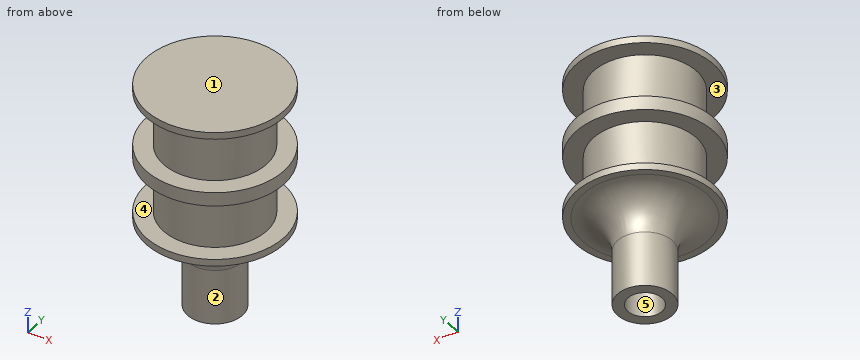
```python
from build123d import *

# Parameters (mm, degrees)
CROQUIS1_R              = 10
SALIENTE_EXTRUIR1_DEPTH = 5
CROQUIS2_R              = 10
CROQUIS2_R_2            = 7.5
CORTAR_EXTRUIR1_DEPTH   = 4
CROQUIS3_R              = 4
SALIENTE_EXTRUIR2_DEPTH = 13
CROQUIS4_R              = 2.5
CORTAR_EXTRUIR2_DEPTH   = 8
REDONDEO1_R             = 5


with BuildPart() as part:
    # Croquis1 → Saliente-Extruir1 (new, symmetric)
    with BuildSketch(Plane(origin=(0, 0, 0), x_dir=(0, 1, 0), z_dir=(0, 0, 1))):
        with Locations(Location((0, 0, 0), (0, 0, 270))):
            Circle(CROQUIS1_R)
    extrude(amount=SALIENTE_EXTRUIR1_DEPTH, both=True)

    # Croquis2 → Cortar-Extruir1 (cut, symmetric)
    with BuildSketch(Plane(origin=(0, 0, 0), x_dir=(0, 1, 0), z_dir=(0, 0, 1))):
        with Locations(Location((0, 0, 0), (0, 0, 270))):
            Circle(CROQUIS2_R)
        with Locations(Location((0, 0, 0), (0, 0, 270))):
            Circle(CROQUIS2_R_2, mode=Mode.SUBTRACT)
    extrude(amount=CORTAR_EXTRUIR1_DEPTH, both=True, mode=Mode.SUBTRACT)

    # Simetría2: part across plane


with BuildPart() as part_1:
    add(part.part)
    add(part.part.mirror(Plane.XY.offset(5)))

    # Croquis3 → Saliente-Extruir2 (add)
    with BuildSketch(Plane(origin=(0, 0, -5), x_dir=(-1, 0, 0), z_dir=(0, 0, -1))):
        with Locations(Location((0, 0, 0), (0, 0, 180))):
            Circle(CROQUIS3_R)
    extrude(amount=SALIENTE_EXTRUIR2_DEPTH)

    # Croquis4 → Cortar-Extruir2 (cut)
    with BuildSketch(Plane(origin=(0, 0, -18), x_dir=(-1, 0, 0), z_dir=(0, 0, -1))):
        Circle(CROQUIS4_R)
    extrude(amount=-CORTAR_EXTRUIR2_DEPTH, mode=Mode.SUBTRACT)

    # Redondeo1
    redondeo1_edges = [part_1.edges().sort_by_distance(p)[0] for p in [
        (-4, 0, -5),
    ]]
    fillet(redondeo1_edges, radius=REDONDEO1_R)


solid = part_1.part
```
Work out the finished part from the listing and answer in its coordinate system (mm). Face numbers are marked on the shaded views. A direction names the side the tool comes from. Give positions to 0.01 mm unless a question says otherwise; leave off trailing zeros. Loops run counter-clockwise (first coordinate to the right, second up) from the corner with the lowest first, then second, coordinate; pieces in that order, holes last. Notation, with made-up numbers: M -29.75,-17 L 13.25,-17 A17 cw 13.25,-4 Z; hole C 69,-33.75 d5. An arc over 180 degrees is marked long. One line per item, written item: value. Start each with the question number.
1. Find section D-D (z = 2.5). Give the vertices of the cut face in (x, y), and give its area (3 significant figures).
2. Find section C-C (z = -12.5). Give the vertices of the cut face in (x, y).
3. Each of these flat-tipped pins is pushed along its axis until it touches: P1, Ø4.5, axis at x = 0, y = 0, coming from the -Z side; P2, Ø6, axis at x = -4.5, y = -3, coming from the -Z side; P3, Ø12, axis at x = 6.5, z = -3, coming from the -Y side; P4, Ø2, axis at x = 6, y = -1.5, coming from the -Z side. Where does it stop, or does it pass through?
4. Which of the six approach directions +Z, -Z, +X, -X, +Y, -Y give full straight-line access (tool end or side, diameter ignored) to the marked faces 4 and 5?
5. Determine the mould class of the marked faces 1, 2 and 3 for opening direction Z: released by +Z, released by -Z, zero draft, split by the parting line, or undercut.
6. Find the intervals of material crossed by probe 1 along Z at (x, y) = (-5.5, -6.75); probe 2 along Y at (x, z) = (0, -11.75); probe 3 along Z at (x, y) = (7.25, -2.75), in increasing order.
Reported:
1. outline: C 0,0 d15
1. area: 177 mm²
2. outline: C 0,0 d8; hole C 0,0 d5
3. P1: stops at z = -10
3. P2: stops at z = -18
3. P3: stops at y = -9.98
3. P4: stops at z = -6.77
4. face 4: none
4. face 5: -Z
5. face 1: released by +Z
5. face 2: zero draft
5. face 3: undercut
6. probe 1: z = -5.01 to -4, 4 to 6, 14 to 15
6. probe 2: y = -4 to -2.5, 2.5 to 4
6. probe 3: z = -5.16 to -4, 4 to 6, 14 to 15
